Can you work these out from the model? Positions are in its coordinate system, mm. Coordinates: 2 decimals unless noted, no trailing zeros. Write each loop counter-clockwise with the first axis right and the second up, starting at its lowest first coordinate (ties: lowest second). Pieces come first, ordered by that corner, then holes.
```python
from build123d import *

# Parameters (mm, degrees)
SKETCH1_W           = 200
SKETCH1_H           = 200
BOSS_EXTRUDE1_DEPTH = 250
FILLET1_R           = 10
SHELL1_START        = -51.838440111
SHELL1_OUTLINE_W    = 230
SHELL1_OUTLINE_H    = 180
SHELL1_DEPTH        = 180
CUT_EXTRUDE1_REACH  = 305.662
FILLET2_R           = 5
CUT_EXTRUDE2_REACH  = 305.662
SKETCH3_R           = 20


# Read off the part's stored shape, not the designer's step: Shell1
with BuildPart() as part:
    # Sketch1 → Boss-Extrude1 (new body)
    with BuildSketch(Plane(origin=(0, 0, 0), x_dir=(1, 0, 0), z_dir=(0, 1, 0))):
        with Locations((38.161559889, 3.064066852)):
            Rectangle(SKETCH1_W, SKETCH1_H)
    extrude(amount=BOSS_EXTRUDE1_DEPTH)

    # Fillet1
    fillet1_edges = [part.edges().sort_by_distance(p)[0] for p in [
        (138.161559889, 250, -3.064066852),
        (38.161559889, 250, -103.064066852),
        (-61.838440111, 250, -3.064066852),
        (-61.838440111, 125, -103.064066852),
        (138.161559889, 125, -103.064066852),
        (138.161559889, 125, 96.935933148),
        (-61.838440111, 125, 96.935933148),
        (38.161559889, 250, 96.935933148),
    ]]
    fillet(fillet1_edges, radius=FILLET1_R)

    # Shell1 outline → Shell1 (cut)
    with BuildSketch(Plane.YZ.offset(SHELL1_START)):
        with Locations((125, -3.064066852)):
            Rectangle(SHELL1_OUTLINE_W, SHELL1_OUTLINE_H)
    extrude(amount=SHELL1_DEPTH, mode=Mode.SUBTRACT)

    # Sketch2 → Cut-Extrude1 (cut, up to next)
    with BuildSketch(Plane(origin=(0, 250, 0), x_dir=(1, 0, 0), z_dir=(0, 1, 0)), mode=Mode.PRIVATE) as cut_extrude1_sk1:
        with BuildLine():
            Line((40.661559889, 20.564066852), (40.661559889, -14.435933148))
            ThreePointArc((40.661559889, -14.435933148), (38.161559889, -16.935933148), (35.661559889, -14.435933148))
            Line((35.661559889, -14.435933148), (35.661559889, 20.564066852))
            ThreePointArc((35.661559889, 20.564066852), (38.161559889, 23.064066852), (40.661559889, 20.564066852))
        make_face()
    cut_extrude1_tool1 = extrude(cut_extrude1_sk1.sketch, amount=-CUT_EXTRUDE1_REACH, mode=Mode.PRIVATE) & part.part
    add(cut_extrude1_tool1.solids().sort_by_distance((38.16156, 250, -3.064067))[0], mode=Mode.SUBTRACT)

    # Fillet2
    fillet2_edges = [part.edges().sort_by_distance(p)[0] for p in [
        (38.161559889, 250, -23.064066852),
        (35.661559889, 250, -3.064066852),
        (38.161559889, 250, 16.935933148),
        (40.661559889, 250, -3.064066852),
    ]]
    fillet(fillet2_edges, radius=FILLET2_R)

    # Sketch3 → Cut-Extrude2 (cut, up to next)
    with BuildSketch(Plane(origin=(0, 0, 0), x_dir=(-1, 0, 0), z_dir=(0, -1, 0)), mode=Mode.PRIVATE) as cut_extrude2_sk1:
        with Locations(Location((-38.161559889, 3.064066852, 0), (0, 0, 90))):
            Circle(SKETCH3_R)
    cut_extrude2_tool1 = extrude(cut_extrude2_sk1.sketch, amount=-CUT_EXTRUDE2_REACH, mode=Mode.PRIVATE) & part.part
    add(cut_extrude2_tool1.solids().sort_by_distance((38.16156, 0, -3.064067))[0], mode=Mode.SUBTRACT)


solid = part.part
```
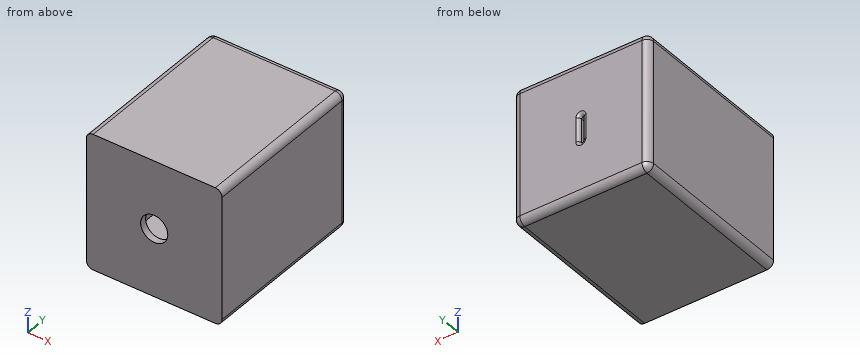
1. If we section it at C-C, the plane x = -15: List the corners of the cut face in (y, z) for me, plus the area to 3 significant figures.
2. If we section it at D-D, the plane x = 52: List the corners of the cut face in (y, z) for me, plus the area to 3 significant figures.
3. I'm going to push a flat-ended pin straight in: P1, Ø5.5, axis at y = 241.5, z = -7.5, coming from the +X side. Where does the tip first touch, or does it pass through?
4. If we section it at A-A, the plane z = -49: List the corners of the cut face in (x, y) for me.
5. If we section it at B-B, the plane y = 173: List the corners of the cut face in (x, z) for me, plus the area to 3 significant figures.
6. If I drill on L1, parallel to X at y = 116, z = -47; L2, parallel to Y at x = 93, z = -1.5; L3, parallel to Z at x = 33, y = 195, over which ranges is the centre line in solid material (lowest first)?
Answers:
1. outline: (0, -103.06) - (240, -103.06) arc R10 ccw to (250, -93.06) - (250, 86.94) arc R10 ccw to (240, 96.94) - (0, 96.94) - close; hole (10, -93.06) - (240, -93.06) - (240, 86.94) - (10, 86.94) - close
1. area: 8,560 mm2
2. outline: (0, -103.06) - (240, -103.06) arc R10 ccw to (250, -93.06) - (250, 86.94) arc R10 ccw to (240, 96.94) - (0, 96.94) - (0, 11.38) - (10, 11.38) - (10, 86.94) - (240, 86.94) - (240, -93.06) - (10, -93.06) - (10, -17.5) - (0, -17.5) - close
2. area: 8,270 mm2
3. P1: stops at x = 138.16
4. outline: (-61.84, 0) - (138.16, 0) - (138.16, 240) arc R10 ccw to (128.16, 250) - (-51.84, 250) arc R10 ccw to (-61.84, 240) - close; hole (-51.84, 10) - (128.16, 10) - (128.16, 240) - (-51.84, 240) - close
5. outline: (-61.84, -93.06) arc R10 ccw to (-51.84, -103.06) - (128.16, -103.06) arc R10 ccw to (138.16, -93.06) - (138.16, 86.94) arc R10 ccw to (128.16, 96.94) - (-51.84, 96.94) arc R10 ccw to (-61.84, 86.94) - close; hole (-51.84, -93.06) - (128.16, -93.06) - (128.16, 86.94) - (-51.84, 86.94) - close
5. area: 7,510 mm2
6. L1: x = -61.84 to -51.84, 128.16 to 138.16
6. L2: y = 0 to 10, 240 to 250
6. L3: z = -103.06 to -93.06, 86.94 to 96.94
